Geometry: final body of the model. Coordinates: model frame, mm. A direction names the side the tool comes from. Give positions to 0.01 mm unless a question says otherwise; leave off trailing zeros. Write each loop counter-clockwise with the first axis right and the second up, starting at its lowest first coordinate (ties: lowest second). Pieces come first, ordered by that corner, then holes. Notation, with made-up numbers: M 22,-38.75 L 30,-38.75 A15 ccw 30,-30.75 Z; hole C 82,10 d8. An arc over 180 degrees is marked long. Answer as a JSON object with one key per item and string values.
Autodesk Inventor part; units mm, degrees
ref_plane "YZ Plane" through (0, 0, 0) normal (1, 0, 0) x (0, 1, 0)
ref_plane "XZ Plane" through (0, 0, 0) normal (0, 1, 0) x (-1, 0, 0)
ref_plane "XY Plane" through (0, 0, 0) normal (0, 0, 1) x (1, 0, 0)
sketch "Sketch19" plane through (0, 0, 0) normal (1, 0, 0) x (0, 1, 0)
  line L0 (0, 0) -> (14.81, 0) construction
  line L1 (0, 0) -> (0, 4.6) construction
  line L2 (0, 29.5) -> (1, 29.5)
  line L3 (1, 29.5) -> (1, 40.5)
  line L4 (1, 40.5) -> (0, 40.5)
  line L5 (0, 40.5) -> (0, 45)
  line L6 (0, 45) -> (12.5, 45)
  line L7 (12.5, 45) -> (12.5, 30)
  line L8 (12.5, 30) -> (4.5, 30)
  line L9 (4.5, 30) -> (4.5, 29)
  line L10 (4.5, 29) -> (3.5, 29)
  line L11 (3.5, 29) -> (3.5, 5.6)
  line L12 (3.5, 5.6) -> (0.5, 5.6)
  line L13 (0.5, 5.6) -> (0.5, 4.6)
  line L14 (0.5, 4.6) -> (0, 4.6)
  line L15 (0, 4.6) -> (0, 29.5)
  dimension "d90" = 0.5
  dimension "d91" = 5.6
  dimension "d92" = 1
  dimension "d93" = 29.5
  dimension "d94" = 40.5
  dimension "d95" = 45
  dimension "d96" = 1
  dimension "d97" = 1
  dimension "d99" = 30
  dimension "d100" = 1
  dimension "d101" = 8
  dimension "d103" = 3
revolve "Revolution2" add sketch "Sketch19" angle 360 about axis through (0, 0, 0) along (0, 1, 0)
sketch "Sketch20" plane through (0, 12.5, 0) normal (0, 1, 0) x (1, 0, 0)
  circle A0 centre (0, 0) radius 35 construction
  circle A1 centre (35, 0) radius 1.75
  dimension "d104" = 70
  dimension "d105" = 3.5
extrude "Extrusion18" cut sketch "Sketch20" against normal through all
sketch "Sketch21" plane through (0, 1, 0) normal (0, -1, 0) x (1, 0, 0)
  line L0 (32.1, 2.9) -> (37.9, 2.9)
  line L1 (37.9, 2.9) -> (37.9, -2.9)
  line L2 (37.9, -2.9) -> (32.1, -2.9)
  line L3 (32.1, -2.9) -> (32.1, 2.9)
  circle A0 centre (35, 0) radius 1.75
  line L4 (32.1, 2.9) -> (37.9, -2.9) construction
  line L5 (37.9, 2.9) -> (32.1, -2.9) construction
  point P0 (0, 0)
  dimension "d108" = 5.8
  dimension "d109" = 5.8
extrude "Extrusion19" cut sketch "Sketch21" against normal blind 3 contours L0 L1 L2 L3 | A0
pattern_circular "Circular Pattern3" count 6 over 360 about axis through (0, 6.25, 0) along (0, 1, 0) of "Extrusion19", "Extrusion18"
sketch "Sketch22" plane through (0, 12.5, 0) normal (0, 1, 0) x (1, 0, 0)
  line L0 (-12.7, 36.27) -> (12.7, 36.27)
  line L1 (12.7, 36.27) -> (12.7, 33.73)
  line L2 (12.7, 33.73) -> (-12.7, 33.73)
  line L3 (-12.7, 33.73) -> (-12.7, 36.27)
  line L4 (-12.7, 36.27) -> (12.7, 33.73) construction
  line L5 (12.7, 36.27) -> (-12.7, 33.73) construction
  line L6 (0, 35) -> (0, 0) construction
  dimension "d115" = 35
  dimension "d116" = 25.4
  dimension "d117" = 2.54
extrude "Extrusion20" cut sketch "Sketch22" against normal through all
properties part number "Wrist_planetary"
1) Contact query for flat-ended pins moving along their axis: P1, Ø3, axis at x = 17.5, z = -30.31, coming from the -Y side; P2, Ø1, axis at y = 6.5, z = -32.5, coming from the -X side; P3, Ø2.5, axis at x = 17, z = 30.5, coming from the -Y side; P4, Ø12, axis at x = -34, z = -23.5, coming from the -Y side. Output: stop coordinate, or through.
Geometry check:
{"P1": "passes through", "P2": "stops at x = -31.64", "P3": "stops at y = 4", "P4": "stops at y = 0"}
2) Cut plane D-D on z = -19. Return loops of the section in (x, y).
Geometry check:
{"outline": "M -40.79,0 L -35.77,0 L -35.77,1 L -22.57,1 L -22.57,0 L 22.57,0 L 22.57,1 L 35.77,1 L 35.77,0 L 40.79,0 L 40.79,12.5 L 23.22,12.5 L 23.22,4.5 L 21.91,4.5 L 21.91,3.5 L -21.91,3.5 L -21.91,4.5 L -23.22,4.5 L -23.22,12.5 L -40.79,12.5 Z"}
3) Line query: line 1 (X direction, y = 2.65, z = 0); line 2 (X direction, y = 0.3, z = 0); line 3 (X direction, y = 0.5, z = -25). Output: solid intervals per line, ascending. Write a range as from..to.
Geometry check:
{"line 1": "x = -45..-37.9, -32.1..-5.6, 5.6..32.1, 37.9..45", "line 2": "x = -45..-40.5, -29.5..-4.6, 4.6..29.5, 40.5..45", "line 3": "x = -37.42..-31.86, -15.66..15.66, 31.86..37.42"}
4) Cut plane C-C on x = -35. Return loops of the section in (y, z).
Geometry check:
{"outline": "M 0,-28.28 L 12.5,-28.28 L 12.5,-1.75 L 4,-1.75 L 4,-2.9 L 1,-2.9 L 1,-20.38 L 0,-20.38 Z; M 0,20.38 L 1,20.38 L 1,2.9 L 4,2.9 L 4,1.75 L 12.5,1.75 L 12.5,28.28 L 0,28.28 Z"}
5) Set-up query: faces 3 (the flat face through (12.7, 7, -35)), 4 (the flat face through (-19, 4, -29)), 5 (the flat face through (5, 0.5, 0)). Return all of +Z, -Z, +X, -X, +Y, -Y with unobstructed straight access to the full face (end or side cutting, diameter ignored); none if empty.
Geometry check:
{"face 3": "+Y, -Y", "face 4": "-Y", "face 5": "+Y"}
6) Pull-direction query (X, two-part tool) for faces 1 (the flat face through (18.99, 2.48, -32.8)), 2 (the cylindrical face through (-39.923, 6.338, 20.765)); classes: pulls with the +X half, pulls with the -X half, needs draft (parallel to the pull), parting line crosses it, or undercut.
Geometry check:
{"face 1": "undercut", "face 2": "parting line crosses it"}
7) Cut plane A-A on x = 0. Give the number of separate pieces and of enclosed holes in the cut face, and give its area (3 significant figures).
Geometry check:
{"separate pieces": "3", "enclosed holes": "0", "area": "498 mm2"}
